from build123d import *

# Parameters (mm, degrees)
SKETCH1_W                = 762
SKETCH1_H                = 762
BOSS_EXTRUDE1_DEPTH      = 139.7
BOSS_EXTRUDE2_DEPTH      = 101.6
BOSS_EXTRUDE4_DEPTH      = 381
BOSS_EXTRUDE4_DEPTH_BACK = 381


with BuildPart() as part:
    # Sketch1 → Boss-Extrude1 (new body)
    with BuildSketch(Plane(origin=(0, 0, 0), x_dir=(1, 0, 0), z_dir=(0, 1, 0))):
        with Locations((0, -1447.8)):
            Rectangle(SKETCH1_W, SKETCH1_H)
        Polygon((381, -977.9), (-381, -977.9), (-977.9, -977.9), (-1066.8, -1066.8), (-381, -1066.8), (381, -1066.8), (1066.8, -1066.8), (977.9, -977.9), align=None)
    extrude(amount=BOSS_EXTRUDE1_DEPTH)

    # Sketch1_10 → Boss-Extrude2 (add)
    with BuildSketch(Plane(origin=(0, 0, 0), x_dir=(1, 0, 0), z_dir=(0, 1, 0))):
        with BuildLine():
            Line((-977.9, -977.9), (977.9, -977.9))
            Line((977.9, -977.9), (215.526146906, -215.526146906))
            ThreePointArc((215.526146906, -215.526146906), (0, -304.8), (-215.526146906, -215.526146906))
            Line((-215.526146906, -215.526146906), (-977.9, -977.9))
        make_face()
    extrude(amount=BOSS_EXTRUDE2_DEPTH)

    # Sketch10 → Boss-Extrude4 (add, two sides: drawn at the far end of the back side and taken through both)
    with BuildSketch(Plane(origin=(0, 0, 0), x_dir=(0, 0, -1), z_dir=(1, 0, 0)).offset(-BOSS_EXTRUDE4_DEPTH_BACK)):
        Polygon((-977.9, 101.6), (-977.9, 139.7), (-838.2, 101.6), align=None)
    extrude(amount=BOSS_EXTRUDE4_DEPTH + BOSS_EXTRUDE4_DEPTH_BACK)


solid = part.part
Here's how the part is built. I have some questions about the finished solid (model axes, mm). A direction names the side the tool comes from. Round coordinates to 2 decimals unless told otherwise and drop trailing zeros. Loops run counter-clockwise (first coordinate to the right, second up) from the corner with the lowest first, then second, coordinate; pieces in that order, holes last. Notation, with made-up numbers: (21, -4.5) - (28, -4.5) arc R25 cw to (28, 33.5) - close; hole circle Ø10 at (80, 72). An arc over 180 degrees is marked (long way). One line per question, with ' | ' between items. Start each with the question number.
Q1. Please list where these lines run through material, in increasing order: line 1 (Y direction, x = -443.5, z = 929.5); line 2 (X direction, y = 96.5, z = 1169.5); line 3 (Z direction, x = -10, y = 12.5). Write a range as [from, to].
Q2. I want a section at A-A (y = 27.5). Write out the boundary of the cut face in (x, z).
Q3. I want a section at C-C (z = 1032). Write out the boundary of the cut face in (x, y), then the cut area to 3 significant figures.
Q4. Will these pins go through, and if not, where does the flat tip stop? pin 1 (10 mm diameter, centred on y = 103, z = 520, fed in from +X); pin 2 (5 mm diameter, centred on y = 47, z = 788, fed in from +X); pin 3 (1 mm diameter, centred on x = -480.5, y = 68.5, fed in from +Z); pin 4 (4 mm diameter, centred on x = -14.5, z = 1487, fed in from -Y).
Q5. We'd pull the mould along X, two halves only. Please class faces 1 (the cylindrical face through (3.35, 50.09, 304.78)), 2 (the flat face through (719, 69, 1066.8)), 3 (the flat face through (381, 69, 1453)): +X half, -X half, draft (parallel to the pull), parting line (faces both ways), or undercut.
Q6. I want a section at D-D (z = 1551.5). Write out the boundary of the cut face in (x, y).
Q7. I want a section at B-B (x = 917). Write out the boundary of the cut face in (y, z).
Q8. For faces 4 (the flat face through (647, 53, 647)), 5 (the flat face through (-381, 69, 1453)), which set-ups out of +Z, -Z, +X, -X, +Y, -Y let a thin tool reach every point of the face, with its end or its side?
Response values:
1) line 1: y = [0, 101.6] | line 2: x = [-381, 381] | line 3: z = [304.64, 1828.8]
2) outline: (-1066.8, 1066.8) - (-215.53, 215.53) arc R304.8 cw to (215.53, 215.53) - (1066.8, 1066.8) - (381, 1066.8) - (381, 1828.8) - (-381, 1828.8) - (-381, 1066.8) - close
3) outline: (-1032, 0) - (1032, 0) - (1032, 139.7) - (-1032, 139.7) - close | area: 288,000 mm²
4) pin 1: stops at x = 524.8 | pin 2: stops at x = 790.5 | pin 3: stops at z = 1066.8 | pin 4: stops at y = 0
5) face 1: undercut | face 2: draft | face 3: +X half
6) outline: (-381, 0) - (381, 0) - (381, 139.7) - (-381, 139.7) - close
7) outline: (0, 917) - (101.6, 917) - (101.6, 977.9) - (139.7, 977.9) - (139.7, 1066.8) - (0, 1066.8) - close
8) face 4: -Z, +X, +Y, -Y | face 5: +Z, -X, +Y, -Y
